Design review of the part built by this model. Coordinates are the model's own, in mm. Face numbers are marked on the shaded views. A direction names the side the tool comes from. Give positions to 0.01 mm unless a question says otherwise; leave off trailing zeros. Order: outer loops, then holes, each group sorted by start corner. A loop starts at its lowest first (then second) coordinate and runs counter-clockwise, first axis right, second up. Notation, with made-up numbers: (-17, -10.75) -> (20, -10.75) arc R32 ccw to (20, 16.25) -> close; hole circle Ø8 at (-23.5, -34). An arc over 180 degrees is marked (long way). One line per item, written item: value.
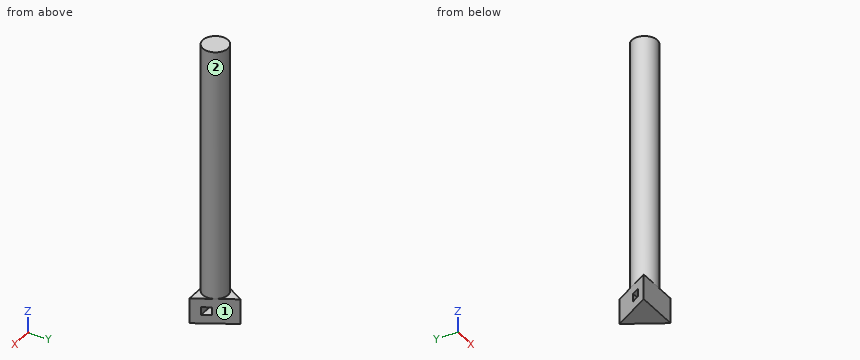
from build123d import *

# Parameters (mm, degrees)
PAD_DEPTH    = 8
SKETCH002_W  = 2.5
SKETCH002_H  = 2.5
POCKET_DEPTH = 12.929203
SKETCH001_R  = 4
PAD001_DEPTH = 80


with BuildPart() as part:
    # Sketch → Pad (new body)
    with BuildSketch(Plane.XY):
        Polygon((-6.928203, -4), (0, 8), (6.928203, -4), align=None)
    extrude(amount=PAD_DEPTH)

    # Sketch002 (on DatumPlane) → Pocket (cut, through all)
    with BuildSketch(Plane(origin=(6, 0, 4), x_dir=(0, 1, 0), z_dir=(1, 0, 0))):
        Rectangle(SKETCH002_W, SKETCH002_H)
    extrude(amount=-POCKET_DEPTH, mode=Mode.SUBTRACT)

    with BuildSketch(Plane.XY.offset(8)):
        Circle(SKETCH001_R)
    extrude(amount=PAD001_DEPTH)


solid = part.part
Item 1: Clearance check with flat-ended pins moving along their axes: P1, Ø1.8, axis at x = 1, y = 4, coming from the +Z side; P2, Ø1.8, axis at x = 5, y = 0, coming from the +Z side; P3, Ø3, axis at x = 5, y = 4, coming from the -Z side; P4, Ø2, axis at y = -1, z = 56, coming from the -X side. State where each tip first meets the part, or that it passes through.
Returned:
P1: z = 88
P2: z = 8
P3: through
P4: x = -4
Item 2: Add section D-D on z = 56. Give the boundary of the cut face in (x, y), plus the area to 3 significant figures.
Returned:
outline: circle Ø8 at (0, 0)
area: 50.3 mm²
Item 3: Add section B-B on z = 7. Give the boundary of the cut face in (x, y), plus the area to 3 significant figures.
Returned:
outline: (-6.93, -4) -> (6.93, -4) -> (0, 8) -> close
area: 83.1 mm²
Item 4: Add section A-A on y = 0. Give the boundary of the cut face in (x, z).
Returned:
outline: (-4.62, 0) -> (4.62, 0) -> (4.62, 2.75) -> (-4.62, 2.75) -> close; (-4.62, 5.25) -> (4.62, 5.25) -> (4.62, 8) -> (4, 8) -> (4, 88) -> (-4, 88) -> (-4, 8) -> (-4.62, 8) -> close
Item 5: Add section C-C on y = 6.5. Give the boundary of the cut face in (x, z), plus the area to 3 significant figures.
Returned:
outline: (-0.87, 0) -> (0.87, 0) -> (0.87, 8) -> (-0.87, 8) -> close
area: 13.9 mm²
Item 6: Machinability: for the marked faces 1 and 2, which of the approach directions +Z, -Z, +X, -X, +Y, -Y give a long, thin tool a straight path to every point of the face, cutting with its end or side? Answer none if there is none.
Returned:
face 1: +Z, -Z, +X, +Y
face 2: +Z
Item 7: To check wall thickness, follow line 1 along Z through (x, y) = (4.25, -1); line 2 along Z through (x, y) = (0, 1); line 3 along Y through (x, z) = (2, 17). State the ranges of each line that lie inside material, in increasing order. Write a range as from..to.
Returned:
line 1: 0..2.75, 5.25..8
line 2: 0..2.75, 5.25..88
line 3: -3.46..3.46
